```python
from build123d import *

# Parameters (mm, degrees)
SKETCH1_W           = 25.4
SKETCH1_H           = 25.4
SKETCH1_W_2         = 19.05
SKETCH1_H_2         = 19.05
BOSS_EXTRUDE1_DEPTH = 128.27
SKETCH2_W           = 46.765463489
SKETCH2_H           = 12.7
CUT_EXTRUDE1_DEPTH  = 12.7
SKETCH4_R           = 3.3734375
CUT_EXTRUDE2_DEPTH  = 132.37596013


with BuildPart() as part:
    # Sketch1 → Boss-Extrude1 (new body)
    with BuildSketch(Plane(origin=(0, 0, 0), x_dir=(1, 0, 0), z_dir=(0, 1, 0))):
        Rectangle(SKETCH1_W, SKETCH1_H)
        Rectangle(SKETCH1_W_2, SKETCH1_H_2, mode=Mode.SUBTRACT)
    extrude(amount=BOSS_EXTRUDE1_DEPTH)

    # Sketch2 → Cut-Extrude1 (cut)
    with BuildSketch(Plane(origin=(0, 0, -12.7), x_dir=(-1, 0, 0), z_dir=(0, 0, -1))):
        with Locations((18.302731745, 44.45)):
            Rectangle(SKETCH2_W, SKETCH2_H)
    extrude(amount=-CUT_EXTRUDE1_DEPTH, mode=Mode.SUBTRACT)

    # Sketch4 → Cut-Extrude2 (cut, through all)
    with BuildSketch(Plane(origin=(12.7, 0, 0), x_dir=(0, 0, -1), z_dir=(1, 0, 0))):
        with Locations((0, 115.57)):
            Circle(SKETCH4_R)
        with Locations((0, 12.7)):
            Circle(SKETCH4_R)
    extrude(amount=-CUT_EXTRUDE2_DEPTH, mode=Mode.SUBTRACT)


solid = part.part
```
Part model, mm, in its own coordinate system. A direction names the side the tool comes from. Round coordinates to 2 decimals unless told otherwise and drop trailing zeros. Loops run counter-clockwise (first coordinate to the right, second up) from the corner with the lowest first, then second, coordinate; pieces in that order, holes last.
Item 1: Cut at A-A, the plane x = 2.75. Give the cut face in (y, z) (3 decimals), then the cut area to 3 significant figures.
Item 2: Drop flat-ended pins along their axis: P1, Ø1.6, axis at y = 42, z = -10.5, coming from the -X side; P2, Ø1, axis at x = -11.5, y = 44, coming from the -Z side. Give the stop position or say it passes through.
Item 3: Cut at B-B, the plane z = 4.5. Give the cut face in (x, y) (3 decimals).
Item 4: Mould opens along Z. For faces 1 (the face through (0, 63, -12.7)), 2 (the face through (11, 128.27, 0)), 3 (the face through (-11.09, 112.277, 0.731)), 4 (the face through (-11.1, 9.4, 0.7)) say: +Z half, -Z half, draft (parallel to the pull), parting line (faces both ways), or undercut.
Item 5: Drill centre lines: line 1 (Y direction, x = 11.9, z = 0); line 2 (X direction, y = 36, z = 7.25) (3 decimals). Where is each one in solid material? Low to high.
Item 6: Cut at D-D, the plane z = -7.25. Give the cut face in (x, y) (3 decimals).
Item 7: Cut at C-C, the plane y = 77.5. Give the cut face in (x, z) (3 decimals), then the cut area to 3 significant figures.
Item 8: 3-axis set-ups, long thin cutter, end or side, ignore diameter. For faces 5 (the face through (11, 0, 0)), 6 (the face through (9.525, 63, 0)), 7 (the face through (-8, 38.1, -11)): which of +Z, -Z, +X, -X, +Y, -Y reach the whole face in a straight line?
A:
1. outline: (0, -12.7) - (38.1, -12.7) - (38.1, -9.525) - (0, -9.525) - close; (0, 9.525) - (128.27, 9.525) - (128.27, 12.7) - (0, 12.7) - close; (50.8, -12.7) - (128.27, -12.7) - (128.27, -9.525) - (50.8, -9.525) - close
1. area: 774 mm2
2. P1: stops at x = 5.08
2. P2: stops at z = 0
3. outline: (-12.7, 0) - (-9.525, 0) - (-9.525, 128.27) - (-12.7, 128.27) - close; (9.525, 0) - (12.7, 0) - (12.7, 128.27) - (9.525, 128.27) - close
4. face 1: -Z half
4. face 2: draft
4. face 3: undercut
4. face 4: undercut
5. line 1: y = 0 to 9.33, 16.07 to 112.2, 118.94 to 128.27
5. line 2: x = -12.7 to -9.525, 9.525 to 12.7
6. outline: (-12.7, 0) - (-9.525, 0) - (-9.525, 38.1) - (-12.7, 38.1) - close; (-12.7, 50.8) - (-9.525, 50.8) - (-9.525, 128.27) - (-12.7, 128.27) - close; (9.525, 0) - (12.7, 0) - (12.7, 128.27) - (9.525, 128.27) - close
7. outline: (-12.7, -12.7) - (12.7, -12.7) - (12.7, 12.7) - (-12.7, 12.7) - close; hole (-9.525, -9.525) - (9.525, -9.525) - (9.525, 9.525) - (-9.525, 9.525) - close
7. area: 282 mm2
8. face 5: +Z, -Z, +X, -X, -Y
8. face 6: +Y, -Y
8. face 7: -Z, -X
